Read the model definition and answer for the solid it produces. Units are mm, in the model's axes. A direction names the side the tool comes from. Coordinates: 2 decimals unless noted, no trailing zeros. Write each loop counter-clockwise with the first axis right and the second up, starting at its lowest first coordinate (ties: lowest second). Pieces come first, ordered by that corner, then holes.
Item 1: Straight lines are drawn through the part: probe 1 along X at (y, z) = (-38, 109); probe 2 along Y at (x, z) = (-576, 94); probe 3 along X at (y, z) = (-15.5, 121). For each, find the intervals that lie inside material, in ascending order.
Item 2: Section C-C (y = -78) is taken. Give the vertices of the cut face in (x, z).
Item 3: Each of these flat-tipped pins is pushed along its axis until it touches: P1, Ø3, axis at x = -545, y = -83, coming from the -Z side; P2, Ø2, axis at y = -83, z = 119.5, coming from the +X side; P3, Ø15, axis at x = -546.18, y = -38.1, coming from the +Z side; P4, Ø6, axis at y = -18.5, z = 125.5, coming from the +X side. Where does it stop, or does it pass through?
Item 4: A tool of negligible diameter and unlimited length cuts with its end or side. For faces 1 (the face through (-495.379, -38, 115)), 2 (the face through (-533.479, -83, 114)), 3 (the face through (-546, -83, 127.247)), 4 (the face through (-501.75, -39.75, 127.14)), 5 (the face through (-549, 0, 113)), from which of +Z, -Z, +X, -X, +Y, -Y can it reach the whole face along a straight path? Write none if from no direction.
Item 5: Section A-A (y = -38.1) is taken. Give the vertices of the cut face in (x, z), then the cut area to 3 significant figures.
Item 6: Section B-B (z = 91.5) is taken. Give the vertices of the cut face in (x, y), then the cut area to 3 significant figures.
from build123d import *

# Parameters (mm, degrees)
F0_W     = 76.2
F0_H     = 76.2
F1_DEPTH = 76.2
F3_D     = 25.4
F4_W     = 25.4
F4_H     = 25.4
F5_DEPTH = 12.7
F6_R     = 12.7
F7_DEPTH = 12.7
F8_R     = 5.08


with BuildPart() as f1:
    # F0 (on Front) → F1 (new body)
    with BuildSketch(Plane.XZ):
        with Locations((-546.1786431313, 114.5474496245)):
            Rectangle(F0_W, F0_H)
    extrude(amount=F1_DEPTH)

    # F3 (through all)
    with Locations(Plane.XY.offset(152.6474496245)):
        with Locations((-546.1786431313, -38.1)):
            Hole(F3_D / 2)

    # F4 (on face) → F5 (join)
    with BuildSketch(Plane.XZ.offset(76.2)):
        with Locations((-546.1786431313, 114.5474496245)):
            Rectangle(F4_W, F4_H)
    extrude(amount=F5_DEPTH)

    # F6 (on face) → F7 (join)
    with BuildSketch(Plane.YZ.offset(-508.0786431313)):
        with Locations((-38.1, 114.5474496245)):
            Circle(F6_R)
    extrude(amount=F7_DEPTH)

    # F8
    f8_edges = [f1.edges().sort_by_distance(p)[0] for p in [
        (-546.178643, -76.2, 152.64745),
        (-584.278643, -38.1, 152.64745),
        (-546.178643, -88.9, 127.24745),
        (-533.478643, -88.9, 114.54745),
        (-546.178643, -88.9, 101.84745),
        (-558.878643, -88.9, 114.54745),
        (-508.078643, -50.8, 114.54745),
        (-495.378643, -50.8, 114.54745),
        (-584.278643, -76.2, 114.54745),
        (-546.178643, -76.2, 76.44745),
        (-508.078643, -76.2, 114.54745),
        (-533.478643, -76.2, 114.54745),
        (-546.178643, -76.2, 127.24745),
        (-558.878643, -76.2, 114.54745),
        (-546.178643, -76.2, 101.84745),
        (-508.078643, -38.1, 152.64745),
        (-508.078643, 0, 114.54745),
        (-508.078643, -38.1, 76.44745),
        (-546.178643, 0, 152.64745),
        (-558.878643, -38.1, 152.64745),
    ]]
    fillet(f8_edges, radius=F8_R)


solid = f1.part
Established:
1. probe 1: x = -584.28 to -558.88, -533.48 to -495.38
1. probe 2: y = -76.2 to 0
1. probe 3: x = -584.28 to -508.08
2. outline: (-560.08, 100.65) - (-532.28, 100.65) - (-532.28, 128.45) - (-560.08, 128.45) - close
3. P1: stops at z = 101.85
3. P2: stops at x = -533.48
3. P3: passes through
3. P4: stops at x = -508.08
4. face 1: +Z, -Z, +X, +Y, -Y
4. face 2: +Z, -Z, +X, -Y
4. face 3: +Z, +X, -X, -Y
4. face 4: +X
4. face 5: +Z, -Z, +X, -X, +Y
5. outline: (-584.28, 76.45) - (-558.88, 76.45) - (-558.88, 147.57) arc R5.08 ccw to (-563.96, 152.65) - (-579.2, 152.65) arc R5.08 ccw to (-584.28, 147.57) - close; (-533.48, 76.45) - (-513.16, 76.45) arc R5.08 ccw to (-508.08, 81.53) - (-508.08, 96.77) arc R5.08 cw to (-503, 101.85) - (-500.46, 101.85) arc R5.08 ccw to (-495.38, 106.93) - (-495.38, 122.17) arc R5.08 ccw to (-500.46, 127.25) - (-503, 127.25) arc R5.08 cw to (-508.08, 132.33) - (-508.08, 147.57) arc R5.08 ccw to (-513.16, 152.65) - (-528.4, 152.65) arc R5.08 ccw to (-533.48, 147.57) - close
5. area: 4,170 mm2
6. outline: (-584.28, -71.12) arc R5.08 ccw to (-579.2, -76.2) - (-513.16, -76.2) arc R5.08 ccw to (-508.08, -71.12) - (-508.08, -5.08) arc R5.08 ccw to (-513.16, 0) - (-584.28, 0) - close; hole circle Ø25.4 at (-546.18, -38.1)
6. area: 5,280 mm2
